from build123d import *

# Parameters (mm, degrees)
SKETCH1_W           = 76
SKETCH1_H           = 47
BOSS_EXTRUDE2_DEPTH = 3
SKETCH2_R           = 1.6
CUT_EXTRUDE1_DEPTH  = 3
SKETCH3_W           = 15
SKETCH3_H           = 18
CUT_EXTRUDE3_DEPTH  = 3


with BuildPart() as part:
    # Sketch1 → Boss-Extrude2 (new body)
    with BuildSketch(Plane(origin=(0, 0, 0), x_dir=(1, 0, 0), z_dir=(0, 1, 0))):
        with Locations((-584.907023411, 237.380936455)):
            Rectangle(SKETCH1_W, SKETCH1_H)
    extrude(amount=BOSS_EXTRUDE2_DEPTH)

    # Sketch2 → Cut-Extrude1 (cut)
    with BuildSketch(Plane(origin=(0, 3, 0), x_dir=(1, 0, 0), z_dir=(0, 1, 0))):
        with Locations((-619.907023411, 257.880936455)):
            Circle(SKETCH2_R)
        with Locations((-549.907023411, 216.880936455)):
            Circle(SKETCH2_R)
    extrude(amount=-CUT_EXTRUDE1_DEPTH, mode=Mode.SUBTRACT)

    # Sketch3 → Cut-Extrude3 (cut)
    with BuildSketch(Plane(origin=(0, 3, 0), x_dir=(1, 0, 0), z_dir=(0, 1, 0))):
        with Locations((-564.407023411, 238.880936455)):
            Rectangle(SKETCH3_W, SKETCH3_H)
    extrude(amount=-CUT_EXTRUDE3_DEPTH, mode=Mode.SUBTRACT)


solid = part.part
Can you work these out from the model? Positions are in its coordinate system, mm. A direction names the side the tool comes from. Coordinates: 2 decimals unless noted, no trailing zeros. Loops run counter-clockwise (first coordinate to the right, second up) from the corner with the lowest first, then second, coordinate; pieces in that order, holes last. Notation, with made-up numbers: M 5,-3 L 58,-3 A15 cw 58,20 Z; hole C 8.25,9.5 d10. An arc over 180 degrees is marked long. Answer as CSV lines item,"result". Start each with the question number.
1. Suppose I cut it at C-C, the plane y = 2.1. List the corners of the cut face in (x, z) for me.
2. Suppose I cut it at B-B, the plane z = -233.5. List the corners of the cut face in (x, y) for me.
3. If I drill on probe 1 along X at (y, z) = (1, -240.5); probe 2 along Z at (x, y) = (-558.5, 0.95); probe 3 along X at (y, z) = (1.8, -217), over which ranges is the centre line in solid material (lowest first)? Write a range as [from, to].
4. Suppose I cut it at A-A, the plane x = -562.5. List the corners of the cut face in (y, z) for me, plus the area to 3 significant figures.
5. Thinking about a two-plate mould opening in Z: for faces 3 (the face through (-585, 1, -260.881)), 4 (the face through (-551.505, 1.521, -216.951)), 5 (the face through (-585, 3, -238)), 6 (the face through (-585, 1, -213.881)), which applies, +Z half, -Z half, draft (parallel to the pull), parting line (faces both ways), or undercut?
6. For pin 1 Ø4 at (x, z) = (-619.91, -257.88) entering from +Y, with a flat end and sliding along its axis, tell me the tip position at first contact or that it passes through.
7. For faces 1 (the face through (-556.907, 2, -239)), 2 (the face through (-546.907, 1, -237)), which set-ups out of +Z, -Z, +X, -X, +Y, -Y let a thin tool reach every point of the face, with its end or its side?
Output:
1,outline,"M -622.91,-260.88 L -546.91,-260.88 L -546.91,-213.88 L -622.91,-213.88 Z; hole C -619.91,-257.88 d3.2; hole M -571.91,-247.88 L -556.91,-247.88 L -556.91,-229.88 L -571.91,-229.88 Z; hole C -549.91,-216.88 d3.2"
2,outline,"M -622.91,0 L -571.91,0 L -571.91,3 L -622.91,3 Z; M -556.91,0 L -546.91,0 L -546.91,3 L -556.91,3 Z"
3,probe 1,"x = [-622.91, -571.91], [-556.91, -546.91]"
3,probe 2,"z = [-260.88, -247.88], [-229.88, -213.88]"
3,probe 3,"x = [-622.91, -551.5], [-548.31, -546.91]"
4,outline,"M 0,-260.88 L 3,-260.88 L 3,-247.88 L 0,-247.88 Z; M 0,-229.88 L 3,-229.88 L 3,-213.88 L 0,-213.88 Z"
4,area,"87.0 mm^2"
5,face 3,"-Z half"
5,face 4,"undercut"
5,face 5,"draft"
5,face 6,"+Z half"
6,pin 1,"stops at y = 3"
7,face 1,"+Y, -Y"
7,face 2,"+Z, -Z, +X, +Y, -Y"
